CAD build for the part. Positions are in the model's coordinates, mm. A direction names the side the tool comes from. Give positions to 0.01 mm unless a question says otherwise; leave off trailing zeros. Order: outer loops, then holes, each group sorted by start corner. A loop starts at its lowest first (then second) coordinate and runs counter-clockwise, first axis right, second up. Notation, with made-up numbers: M 48,87.25 L 82,87.25 A12 ccw 82,98.25 Z; hole C 78.25,24.25 d8. An arc over 180 degrees is marked long. Put each result on its own line as item: value. Start each with the question number.
1) Cut at C-C (x = -25.5). Write the cut outline in (y, z).
2) Cut at B-B (y = 21.5). Write the cut outline in (x, z), and give its area (3 significant figures).
3) Two-plate mould, pull along Y, no slides. Class faces 1 (the face through (-4.4, 20.4, -7)), 2 (the face through (-25.746, -1.421, -3.451)), 3 (the face through (-37.241, 19.994, -3.451)), 4 (the face through (-13.022, 21.338, -3.451)): released by +Y, released by -Y, zero draft, split by the parting line, or undercut.
4) Drill centre lines: line 1 (Y direction, x = 14, z = -4.5); line 2 (Y direction, x = 7.5, z = -5). Where is each one in solid material? Low to high. Write a range as [from, to].
5) Cut at A-A (z = -1). Write the cut outline in (x, y), and give its area (3 significant figures).
6) Tool access for faces 5 (the face through (-4.4, 20.4, 0)), 6 (the face through (-25.3, -0.4, -3.5)): list every direction of +Z, -Z, +X, -X, +Y, -Y with a clear straight run to the whole face (end or side of a thin tool).
7) Pin check, flat tips, straight feed: pin 1 (4 mm diameter, centred on y = -12.5, z = -3, fed in from +X); pin 2 (1 mm diameter, centred on x = 11, y = 17, fed in from +Z). Stop position of each tip, or through.
```python
from build123d import *

# Parameters (mm, degrees)
BOSS_EXTRUDE1_DEPTH = 7


with BuildPart() as part:
    # Sketch1 → Boss-Extrude1 (new body)
    with BuildSketch(Plane.XY):
        with BuildLine():
            Line((-28.84670785, 24.383284156), (2.617804957, 20.332169024))
            ThreePointArc((2.617804957, 20.332169024), (17.738884876, 10.27530843), (18.939530416, -7.845010363))
            ThreePointArc((18.939530416, -7.845010363), (3.206757045, -20.247634658), (-15.588518883, -13.313454812))
            Line((-15.588518883, -13.313454812), (-36.191405321, 10.810147126))
            ThreePointArc((-36.191405321, 10.810147126), (-37.176177413, 20.116777399), (-28.84670785, 24.383284156))
        make_face()
        with BuildLine():
            ThreePointArc((-28.974405652, 23.391471033), (-36.296684217, 19.64086594), (-35.430989766, 11.459583946))
            Line((-35.430989766, 11.459583946), (-14.828103328, -12.664017991))
            ThreePointArc((-14.828103328, -12.664017991), (3.050329872, -19.259945163), (18.015650884, -7.462326931))
            ThreePointArc((18.015650884, -7.462326931), (16.873573419, 9.774073873), (2.490107155, 19.340355901))
            Line((2.490107155, 19.340355901), (-28.974405652, 23.391471033))
        make_face(mode=Mode.SUBTRACT)
    extrude(amount=-BOSS_EXTRUDE1_DEPTH)


solid = part.part
```
Solution:
1. outline: M -1.71,-7 L -0.17,-7 L -0.17,0 L -1.71,0 Z; M 22.94,-7 L 23.95,-7 L 23.95,0 L 22.94,0 Z
2. outline: M -36.24,-7 L -34.86,-7 L -34.86,0 L -36.24,0 Z; M -14.28,-7 L -6.45,-7 L -6.45,0 L -14.28,0 Z
2. area: 64.5 mm²
3. face 1: zero draft
3. face 2: released by -Y
3. face 3: split by the parting line
3. face 4: undercut
4. line 1: [-14.97, -13.57], [13.57, 14.97]
4. line 2: [-19.08, -18], [18, 19.08]
5. outline: M -36.19,10.81 L -15.59,-13.31 A20.5 ccw long 2.62,20.33 L -28.85,24.38 A8.27 ccw Z; hole M -35.43,11.46 L -14.83,-12.66 A19.5 ccw long 2.49,19.34 L -28.97,23.39 A7.27 ccw Z
5. area: 160 mm²
6. face 5: +Z, +X, -X, +Y, -Y
6. face 6: +Z, -Z
7. pin 1: x = 17.61
7. pin 2: z = 0
